Work out the finished part from the listing and answer in its coordinate system (mm). A direction names the side the tool comes from. Coordinates: 2 decimals unless noted, no trailing zeros. Loops run counter-clockwise (first coordinate to the right, second up) from the corner with the lowest first, then second, coordinate; pieces in that order, holes last. Notation, with made-up numbers: M -25.5,28 L 15.5,28 A16 cw 15.5,56 Z; hole C 69.5,-20 d2. An arc over 180 degrees is marked long. Write each question's results on one line, items separated by ' | '.
Autodesk Fusion 360 part; units mm, degrees
sketch "Sketch1" plane through (0, 0, 0) normal (0, 0, 1) x (1, 0, 0)
  circle A0 centre (0, 0) radius 1.8
  circle A1 centre (61, 0) radius 1.8
  circle A2 centre (0, 31) radius 1.8
  circle A3 centre (61, 31) radius 1.8
  line L0 (-3, 34) -> (64, 34)
  line L1 (64, 34) -> (64, -3)
  line L2 (64, -3) -> (-3, -3)
  line L3 (-3, -3) -> (-3, 34)
  dimension "d3" = 61
  dimension "d4" = 31
  dimension "d5" = 3.6
  dimension "d6" = 3
  dimension "d7" = 3
  dimension "d8" = 3
  dimension "d9" = 3
extrude "Extrude1" add sketch "Sketch1" along normal blind 2
sketch "Sketch2" plane through (0, 0, 2) normal (0, 0, 1) x (-1, 0, 0)
  circle A0 centre (0, 0) radius 1.8
  circle A1 centre (-61, 0) radius 1.8
  circle A2 centre (-61, -31) radius 1.8
  circle A3 centre (0, -31) radius 1.8
  line L0 (3, 3) -> (-64, 3)
  line L1 (-64, 3) -> (-64, -34)
  line L2 (-64, -34) -> (3, -34)
  line L3 (3, -34) -> (3, 3)
  circle A4 centre (0, -31) radius 3
  line L4 (-3, -31) -> (-3, -34)
  line L5 (0, -28) -> (3, -28)
  circle A5 centre (-61, -31) radius 3
  line L6 (-61, -28) -> (-64, -28)
  line L7 (-58, -31) -> (-58, -34)
  circle A6 centre (-61, 0) radius 3
  line L8 (-58, 0) -> (-58, 3)
  line L9 (-61, -3) -> (-64, -3)
  circle A7 centre (0, 0) radius 3
  line L10 (-3, 0) -> (-3, 3)
  line L11 (0, -3) -> (3, -3)
extrude "Extrude2" add sketch "Sketch2" along normal blind 2 contours L0 A7 L10 | L0 A6 L8 | L0 L3 A7 | A7 | L0 L1 A6 | A6 | L3 A7 L11 | L1 A6 L9 | L3 A4 L5 | L1 A5 L6 | A4 | L2 L3 A4 | L1 L2 A5 | A5 | L2 A5 L7
equation "d7 = d6"
equation "d8 = d6"
equation "d9 = d6"
1) Which of the six approach directions +Z, -Z, +X, -X, +Y, -Y give full straight-line access (tool end or side, diameter ignored) to faces 1 (the face through (58, 32, 3)), 2 (the face through (-0.119, 1.796, 2.416)), 3 (the face through (-1, 3, 3)), 4 (the face through (2.1, 2.14, 2.99))?
Check result:
face 1: +Z, +Y, -Y | face 2: +Z, -Z | face 3: +Z, +X, -X | face 4: +Z
2) Straight lines are drawn through the part: probe 1 along X at (y, z) = (31, 1.4); probe 2 along Y at (x, z) = (0, 1.5); probe 3 along Y at (x, z) = (61, 3.2). For each, find the intervals that lie inside material, in ascending order. Write a range as [from, to].
Check result:
probe 1: [-3, -1.8], [1.8, 59.2], [62.8, 64] | probe 2: [-3, -1.8], [1.8, 29.2], [32.8, 34] | probe 3: [-3, -1.8], [1.8, 3], [28, 29.2], [32.8, 34]
3) Find section A-A, the plane z = 1.4. Give the vertices of the cut face in (x, y), and give its area (3 significant figures).
Check result:
outline: M -3,-3 L 64,-3 L 64,34 L -3,34 Z; hole C 0,0 d3.6; hole C 0,31 d3.6; hole C 61,0 d3.6; hole C 61,31 d3.6 | area: 2,440 mm^2
4) Find section C-C, the plane y = 10. Give the vertices of the cut face in (x, z), and give its area (3 significant figures).
Check result:
outline: M -3,0 L 64,0 L 64,2 L -3,2 Z | area: 134 mm^2
5) Find section B-B, the plane x = 22.5. Give the vertices of the cut face in (y, z), and give its area (3 significant figures).
Check result:
outline: M -3,0 L 34,0 L 34,2 L -3,2 Z | area: 74.0 mm^2
6) Given pin 1 Ø8 at (x, y) = (7, 25) entering from +Z, flat-ended and moving along its own axis, determine where the tip first touches the part or whether it passes through.
Check result:
pin 1: z = 2
7) For a pull along X with two mould halves and no side action, classify faces 5 (the face through (62, 3, 3)), 6 (the face through (64, 15.8, 1.5)), 7 (the face through (58.86, 2.1, 2.99)) as released by +X, released by -X, zero draft, split by the parting line, or undercut.
Check result:
face 5: zero draft | face 6: released by +X | face 7: undercut
